Autodesk Inventor part; units mm, degrees
ref_plane "YZ Plane" through (0, 0, 0) normal (1, 0, 0) x (0, 1, 0)
ref_plane "XZ Plane" through (0, 0, 0) normal (0, 1, 0) x (-1, 0, 0)
ref_plane "XY Plane" through (0, 0, 0) normal (0, 0, 1) x (1, 0, 0)
sketch "Sketch1" plane through (0, 0, 0) normal (0, 1, 0) x (-1, 0, 0)
  circle A0 centre (0, 0) radius 4.6
  dimension "d0" = 9.2
extrude "Extrusion1" add sketch "Sketch1" along normal blind 1.2
sketch "Sketch2" plane through (0, 1.2, 0) normal (0, 1, 0) x (1, 0, 0)
  line L0 (-3.9837, 0) -> (-1.9919, 3.45)
  line L1 (-1.9919, 3.45) -> (1.9919, 3.45)
  line L2 (1.9919, 3.45) -> (3.9837, 0)
  line L3 (3.9837, 0) -> (1.9919, -3.45)
  line L4 (1.9919, -3.45) -> (-1.9919, -3.45)
  line L5 (-1.9919, -3.45) -> (-3.9837, 0)
  point P0 (0, 0)
  point P1 (0, 0)
  dimension "d3" = 6.9
extrude "Extrusion2" add sketch "Sketch2" along normal blind 3
sketch "Sketch3" plane through (0, 4.2, 0) normal (0, 1, 0) x (1, 0, 0)
  circle A0 centre (0, 0) radius 3.25
  dimension "d6" = 6.5
extrude "Extrusion3" add sketch "Sketch3" along normal blind 1.5
sketch "Sketch4" plane through (0, 0, 0) normal (0, -1, 0) x (1, 0, 0)
  circle A0 centre (0, 0) radius 1.75
  dimension "d9" = 3.5
extrude "Extrusion4" cut sketch "Sketch4" against normal through all
thread "Thread1"
properties part number "H003_Tuerca_M4X5_7"
Here's how the part is built. I have some questions about the finished solid (model axes, mm). A direction names the side the tool comes from. Coordinates: 2 decimals unless noted, no trailing zeros. Loops run counter-clockwise (first coordinate to the right, second up) from the corner with the lowest first, then second, coordinate; pieces in that order, holes last. Notation, with made-up numbers: (-38.5, 30.5) - (-25.5, 30.5) arc R25 cw to (-25.5, 47.5) - close; hole circle Ø7 at (11.5, -9.5). An arc over 180 degrees is marked (long way). Answer as CSV lines item,"result".
Q1. If we section it at D-D, the plane z = -3: Write out the boundary of the cut face in (x, y), and give its area (3 significant figures).
Response:
outline,"(-3.49, 0) - (3.49, 0) - (3.49, 1.2) - (2.25, 1.2) - (2.25, 4.2) - (1.25, 4.2) - (1.25, 5.7) - (-1.25, 5.7) - (-1.25, 4.2) - (-2.25, 4.2) - (-2.25, 1.2) - (-3.49, 1.2) - close"
area,"25.6 mm2"
Q2. If we section it at A-A, the plane x = 0: Write out the boundary of the cut face in (y, z).
Response:
outline,"(0, -4.6) - (1.2, -4.6) - (1.2, -3.45) - (4.2, -3.45) - (4.2, -3.25) - (5.7, -3.25) - (5.7, -1.75) - (0, -1.75) - close; (0, 1.75) - (5.7, 1.75) - (5.7, 3.25) - (4.2, 3.25) - (4.2, 3.45) - (1.2, 3.45) - (1.2, 4.6) - (0, 4.6) - close"
Q3. For faces 4 (the face through (3, 2.7, 1.7)), 5 (the face through (-3, 2.7, 1.7)), 6 (the face through (0, 3, -3.45)), which set-ups out of +Z, -Z, +X, -X, +Y, -Y let a thin tool reach every point of the face, with its end or its side?
Response:
face 4,"+Z, +X, +Y"
face 5,"+Z, -X, +Y"
face 6,"-Z, +X, -X, +Y"
Q4. If we section it at C-C, the plane z = -1.5: Write out the boundary of the cut face in (x, y).
Response:
outline,"(-4.35, 0) - (-0.9, 0) - (-0.9, 5.7) - (-2.88, 5.7) - (-2.88, 4.2) - (-3.12, 4.2) - (-3.12, 1.2) - (-4.35, 1.2) - close; (0.9, 0) - (4.35, 0) - (4.35, 1.2) - (3.12, 1.2) - (3.12, 4.2) - (2.88, 4.2) - (2.88, 5.7) - (0.9, 5.7) - close"
Q5. For pin 1 (3 mm diameter, centred on x = -3, y = 3.5, fed in from +Z); pin 2 (3 mm diameter, centred on y = 3, z = 3, fed in from -X); pin 3 (3 mm diameter, centred on y = 5, z = -1.5, fed in from +X), each with a flat end and sliding along its axis, tell me the tip position at first contact or that it passes through.
Response:
pin 1,"z = 3.45"
pin 2,"x = -3.12"
pin 3,"x = 3.85"
Q6. We'd pull the mould along Z, two halves only. Please class faces 1 (the face through (-2.579, 4.94, -1.978)), 2 (the face through (-3, 2.7, -1.7)), 3 (the face through (1.617, 2.81, -0.67)): pulls with the +Z half, pulls with the -Z half, needs draft (parallel to the pull), parting line crosses it, or undercut.
Response:
face 1,"parting line crosses it"
face 2,"pulls with the -Z half"
face 3,"undercut"
Q7. If we section it at B-B, the plane y = 2.75: Write out the boundary of the cut face in (x, z).
Response:
outline,"(-3.98, 0) - (-1.99, -3.45) - (1.99, -3.45) - (3.98, 0) - (1.99, 3.45) - (-1.99, 3.45) - close; hole circle Ø3.5 at (0, 0)"
Q8. If I drill on L1, parallel to Z at x = 0, y = 3.3; L2, parallel to X at y = 2.15, z = -0.25; L3, parallel to Y at x = -0.5, z = 3.25, over which ranges is the centre line in solid material (lowest first)? Write a range as [from, to].
Response:
L1,"[-3.45, -1.75], [1.75, 3.45]"
L2,"[-3.84, -1.73], [1.73, 3.84]"
L3,"[0, 4.2]"
